Could you check a few things on this model? Use its own coordinates, in mm. Face numbers are marked on the shaded views. A direction names the side the tool comes from. Coordinates: 2 decimals unless noted, no trailing zeros. Order: outer loops, then holes, each group sorted by start corner. A loop starts at its lowest first (then second) coordinate and runs counter-clockwise, first axis right, second up. Notation, with made-up numbers: (-22.75, 78) - (-1.75, 78) arc R31 ccw to (-1.75, 117) - close; hole circle Ø10 at (20, 43). An arc over 180 degrees is marked (long way). Answer as CSV lines item,"result". Start each with the question number.
1. I want a section at A-A, the plane y = -30. List the corners of the cut face in (x, z) for me.
2. I want a section at B-B, the plane z = -34.5. List the corners of the cut face in (x, y) for me, and give its area (3 significant figures).
3. For pin 1 (10 mm diameter, centred on x = 52, z = 45.5, fed in from -Y); pin 2 (12 mm diameter, centred on x = -5.5, y = -77.5, fed in from +Z); pin 3 (15 mm diameter, centred on y = -52, z = -13, fed in from -X); pin 4 (6 mm diameter, centred on x = 53, z = -6, fed in from +Y), each with a flat end and sliding along its axis, tell me the tip position at first contact or that it passes through.
4. Thinking about a two-plate mould opening in Z: for the marked faces 4, 5, 6 and 7, which applies, released by +Z, released by -Z, zero draft, split by the parting line, or undercut?
5. For the marked faces 1, 2 and 3, which set-ups out of +Z, -Z, +X, -X, +Y, -Y let a thin tool reach every point of the face, with its end or its side?
6. I need wall thicknesses on probe 1 along Z at (x, y) = (21.5, -86.5); probe 2 along X at (y, z) = (-65.5, -34.5); probe 3 along X at (y, z) = (-12, 51). Which ranges of each line are inside material? Lowest first, please.
7. I want a section at C-C, the plane x = -42.5. List the corners of the cut face in (y, z) for me, and give its area (3 significant figures).
from build123d import *

# Parameters (mm, degrees)
F1_DEPTH = 150
F2_W     = 100
F2_H     = 20
F3_DEPTH = 25.4


with BuildPart() as f1:
    # F0 (on Front) → F1 (new body)
    with BuildSketch(Plane.XZ):
        Polygon((87.471645, 90), (67.471645, 90), (67.471645, 10), (-37.471645, 10), (-37.471645, -40), (-87.471645, -40), (-87.471645, -90), (87.471645, -90), align=None)
    extrude(amount=F1_DEPTH)

    # F2 (on face) → F3 (join)
    with BuildSketch(Plane(origin=(67.471645, 0, 0), x_dir=(0, -1, 0), z_dir=(-1, 0, 0))):
        with Locations((75, 50)):
            Rectangle(F2_W, F2_H)
    extrude(amount=F3_DEPTH)


solid = f1.part
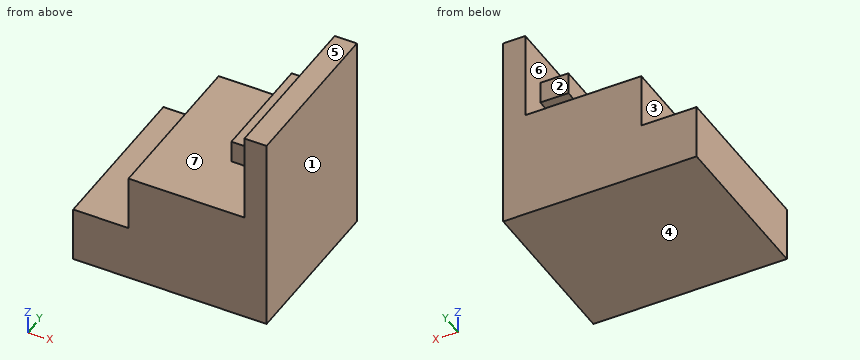
Solved:
1,outline,"(-87.47, -90) - (87.47, -90) - (87.47, 90) - (67.47, 90) - (67.47, 60) - (42.07, 60) - (42.07, 40) - (67.47, 40) - (67.47, 10) - (-37.47, 10) - (-37.47, -40) - (-87.47, -40) - close"
2,outline,"(-37.47, -150) - (87.47, -150) - (87.47, 0) - (-37.47, 0) - close"
2,area,"18,700 mm2"
3,pin 1,"stops at y = -125"
3,pin 2,"stops at z = 10"
3,pin 3,"stops at x = -37.47"
3,pin 4,"stops at y = 0"
4,face 4,"released by -Z"
4,face 5,"released by +Z"
4,face 6,"undercut"
4,face 7,"undercut"
5,face 1,"+Z, -Z, +X, +Y, -Y"
5,face 2,"+Z, -X, +Y"
5,face 3,"+Z, -X, +Y, -Y"
6,probe 1,"z = -90 to 10"
6,probe 2,"x = -37.47 to 87.47"
6,probe 3,"x = 67.47 to 87.47"
7,outline,"(-150, -90) - (0, -90) - (0, -40) - (-150, -40) - close"
7,area,"7,500 mm2"
